Can you work these out from the model? Positions are in its coordinate system, mm. A direction names the side the tool comes from. Round coordinates to 2 decimals unless told otherwise and drop trailing zeros. Answer as CSV lines item,"result".
```python
from build123d import *

# Parameters (mm, degrees)
F0_R     = 10.16
F1_DEPTH = 15.7734
F2_DEPTH = 40.2336
F3_R     = 3.066051


with BuildPart() as f1:
    # F0 (on Front) → F1 (new body)
    with BuildSketch(Plane.XZ):
        with BuildLine():
            ThreePointArc((-18.485138, 27.110208), (-7.646431, 20.535508), (-0.718441, 9.919144))
            ThreePointArc((-0.718441, 9.919144), (1.044836, 0.88042), (-0.158376, -8.249748))
            ThreePointArc((-0.158376, -8.249748), (-7.023149, -19.913542), (-18.485138, -27.110208))
            Line((-18.485138, -27.110208), (30.22916, -13.78093))
            ThreePointArc((30.22916, -13.78093), (40.745902, 0), (30.22916, 13.78093))
            Line((30.22916, 13.78093), (-18.485138, 27.110208))
        make_face()
        with Locations((26.458402, 0)):
            Circle(F0_R, mode=Mode.SUBTRACT)
    extrude(amount=F1_DEPTH)

    # F0 (on Front) → F2 (join)
    with BuildSketch(Plane.XZ):
        with BuildLine():
            ThreePointArc((-0.158376, -8.249748), (1.044836, 0.88042), (-0.718441, 9.919144))
            ThreePointArc((-0.718441, 9.919144), (-7.646431, 20.535508), (-18.485138, 27.110208))
            ThreePointArc((-18.485138, 27.110208), (-56.091598, 0), (-18.485138, -27.110208))
            ThreePointArc((-18.485138, -27.110208), (-7.023149, -19.913542), (-0.158376, -8.249748))
        make_face()
        with BuildLine():
            ThreePointArc((-14.907705, -6.719262), (-41.804098, 0), (-14.907705, 6.719262))
            Line((-14.907705, 6.719262), (-8.855358, 6.719262))
            Line((-8.855358, 6.719262), (-8.855358, -6.719262))
            Line((-8.855358, -6.719262), (-14.907705, -6.719262))
        make_face(mode=Mode.SUBTRACT)
    extrude(amount=F2_DEPTH)

    # F3
    f3_edges = [f1.edges().sort_by_distance(p)[0] for p in [
        (-36.548058, -40.2336, 27.110208),
    ]]
    fillet(f3_edges, radius=F3_R)


solid = f1.part
```
Q1. If I drill on line 1 along X through (y, z) = (-18, 0); line 2 along X through (y, z) = (-3, -3); line 3 along Z through (x, y) = (-22.5, -22), over which ranges is the centre line in solid material (lowest first)? Write a range as [from, to].
Checks:
line 1,"[-56.09, -41.8], [-8.86, 1.06]"
line 2,"[-55.93, -41.49], [-8.86, 16.75], [36.17, 40.43]"
line 3,"[-28.13, -13.38], [13.38, 28.13]"
Q2. We'd pull the mould along X, two halves only. Please class faces 3 (the flat face through (-12, -20, 6.719)), 4 (the flat face through (-39, -40.234, -11)), 5 (the flat face through (-8.855, -20, 0)), 6 (the flat face through (5.53, -7.78, -20.54)): pulls with the +X half, pulls with the -X half, needs draft (parallel to the pull), parting line crosses it, or undercut.
Checks:
face 3,"undercut"
face 4,"needs draft"
face 5,"undercut"
face 6,"pulls with the +X half"
Q3. On a 3-axis mill with a long thin cutter (end or side, diameter ignored), from which of +Z, -Z, +X, -X, +Y, -Y can I reach the whole of each face in a straight line? I mean faces 1 (the flat face through (-12, -20, -6.719)), 2 (the cylindrical face through (40.744, -7.776, -0.261)). Say none if no direction works.
Checks:
face 1,"+Y, -Y"
face 2,"+X, +Y, -Y"
Q4. Imagine slicing it at B-B (y = -6). Count the separate pieces of the cut face and the enclosed holes in it, then the cut area to 3 significant figures.
Checks:
separate pieces,"1"
enclosed holes,"2"
area,"2,960 mm²"
Q5. I'm going to push flat-ended pins straight in: pin 1 Ø1 at (x, y) = (-3.5, -18) entering from +Z; pin 2 Ø2 at (x, y) = (10, -16) entering from -Z; pin 3 Ø1.8 at (x, y) = (-11.5, -21.5) entering from +Z. Where does each tip first touch, or does it pass through?
Checks:
pin 1,"z = 16.23"
pin 2,"z = -19.58"
pin 3,"z = 24.25"
